from build123d import *

# Parameters (mm, degrees)
F0_W     = 53.15
F0_H     = 95.12
F1_DEPTH = 2
F2_R     = 4.5
F3_DEPTH = 36.36


with BuildPart() as f1:
    # F0 (on Top) → F1 (new body)
    with BuildSketch(Plane.XY):
        Rectangle(F0_W, F0_H)
        with BuildLine():
            Line((-22.675, -42.035), (-22.675, -39.625))
            ThreePointArc((-22.675, -39.625), (-19.95, -36.9), (-17.225, -39.625))
            Line((-17.225, -39.625), (-17.225, -42.035))
            ThreePointArc((-17.225, -42.035), (-19.95, -44.76), (-22.675, -42.035))
        make_face(mode=Mode.SUBTRACT)
        with BuildLine():
            ThreePointArc((17.225, -39.625), (19.95, -36.9), (22.675, -39.625))
            Line((22.675, -39.625), (22.675, -42.035))
            ThreePointArc((22.675, -42.035), (19.95, -44.76), (17.225, -42.035))
            Line((17.225, -42.035), (17.225, -39.625))
        make_face(mode=Mode.SUBTRACT)
        with BuildLine():
            Line((-17.225, 42.035), (-17.225, 39.625))
            ThreePointArc((-17.225, 39.625), (-19.95, 36.9), (-22.675, 39.625))
            Line((-22.675, 39.625), (-22.675, 42.035))
            ThreePointArc((-22.675, 42.035), (-19.95, 44.76), (-17.225, 42.035))
        make_face(mode=Mode.SUBTRACT)
        with BuildLine():
            ThreePointArc((17.225, 42.035), (19.95, 44.76), (22.675, 42.035))
            Line((22.675, 42.035), (22.675, 39.625))
            ThreePointArc((22.675, 39.625), (19.95, 36.9), (17.225, 39.625))
            Line((17.225, 39.625), (17.225, 42.035))
        make_face(mode=Mode.SUBTRACT)
    extrude(amount=F1_DEPTH)

    # F2 (on face) → F3 (join)
    with BuildSketch(Plane.XY.offset(2)):
        Circle(F2_R)
    extrude(amount=F3_DEPTH)

    # F4 (on Front) → F5 (revolve)
    with BuildSketch(Plane.XZ):
        with BuildLine():
            Line((0, 38.36), (7.088723, 38.36))
            ThreePointArc((7.088723, 38.36), (17.120894, 57.982844), (0, 71.86))
            Line((0, 71.86), (0, 38.36))
        make_face()
    revolve(axis=Axis((0, 0, 55.11), (0, 0, -1)))


solid = f1.part
Geometry check sheet. Reference: the model listing, model coordinates, mm. A direction names the side the tool comes from. Give positions to 0.01 mm unless a question says otherwise; leave off trailing zeros. Order: outer loops, then holes, each group sorted by start corner. A loop starts at its lowest first (then second) coordinate and runs counter-clockwise, first axis right, second up.
1) Cross-section at A-A (x = -19.95). Record the boundary of the cut face in (y, z).
Results are:
outline: (-47.56, 0) - (-44.76, 0) - (-44.76, 2) - (-47.56, 2) - close; (-36.9, 0) - (36.9, 0) - (36.9, 2) - (-36.9, 2) - close; (44.76, 0) - (47.56, 0) - (47.56, 2) - (44.76, 2) - close
2) Cross-section at B-B (z = 13). Record the boundary of the cut face in (x, y), then the cut area to 3 significant figures.
Results are:
outline: circle Ø9 at (0, 0)
area: 63.6 mm2
3) Draft check along Z on faces 4 (the flat face through (6, 1, 2)), 5 (the flat face through (0, 1, 0)), 6 (the flat face through (-26.575, -1, 1)). Enter one of: released by +Z, released by -Z, zero draft, split by the parting line, or undercut.
Results are:
face 4: undercut
face 5: released by -Z
face 6: zero draft
4) Material ranges on probe 1 along Z at (x, y) = (18.5, -24); probe 2 along Y at (x, z) = (11.5, 52.5); probe 3 along Y at (x, z) = (-1, 35), recorded low to high.
Results are:
probe 1: z = 0 to 2
probe 2: y = -13.06 to 13.06
probe 3: y = -4.39 to 4.39
5) Gauge pin test, flat ends, axial feed: pin 1 (4 mm diameter, centred on x = 7, y = -2, fed in from -Z); pin 2 (6 mm diameter, centred on x = -6, z = 52.5, fed in from +Y); pin 3 (2 mm diameter, centred on x = 4.5, z = 22, fed in from +Y); pin 4 (6 mm diameter, centred on x = -18.5, z = 53.5, fed in from +Y). Record the tip position at first contact, or that the pin passes through.
Results are:
pin 1: stops at z = 0
pin 2: stops at y = 17.19
pin 3: stops at y = 2.83
pin 4: stops at y = 8.09
6) Tool access check on faces 1 (the flat face through (26.575, -1, 1)), 2 (the cylindrical face through (-0.59, 4.46, 19.93)), 3 (the flat face through (-17.225, 41, 1)). Record the directions out of +Z, -Z, +X, -X, +Y, -Y that give a thin tool (end or side, any length) a straight path to the whole face; none if there is none.
Results are:
face 1: +Z, -Z, +X, +Y, -Y
face 2: none
face 3: +Z, -Z
7) Cross-section at C-C (y = -26.5). Record the boundary of the cut face in (x, z) (3 decimals).
Results are:
outline: (-26.575, 0) - (26.575, 0) - (26.575, 2) - (-26.575, 2) - close
